Read the model definition and answer for the solid it produces. Units are mm, in the model's axes. Face numbers are marked on the shaded views. A direction names the side the tool comes from. Give positions to 0.01 mm unless a question says otherwise; leave off trailing zeros. Write each loop counter-clockwise with the first axis right and the second up, starting at its lowest first coordinate (ties: lowest second). Pieces come first, ordered by that corner, then holes. Notation, with made-up numbers: M -32.5,5 L -18.5,5 A23 ccw -18.5,18 Z; hole C 37.25,25.25 d11. An arc over 180 degrees is marked long. Put each result on its own line as item: value.
from build123d import *

# Parameters (mm, degrees)
ENL_V_START             = -10
ENL_V_MAT_EXTRU_1_DEPTH = 10


with BuildPart() as part:
    # Esquisse1 → R_volution1 (revolve)
    with BuildSketch(Plane.XY, mode=Mode.PRIVATE) as r_volution1_sk:
        with BuildLine():
            Line((38.667823993, 0), (38.667823993, 1.585))
            Line((38.667823993, 1.585), (36.667823993, 1.585))
            Line((36.667823993, 1.585), (33.667823993, 4.585))
            Line((33.667823993, 4.585), (33.667823993, 7.5))
            Line((33.667823993, 7.5), (40.667823993, 7.5))
            Line((40.667823993, 7.5), (40.667823993, 1.5))
            Line((40.667823993, 1.5), (47.667823993, 1.5))
            Line((47.667823993, 1.5), (47.667823993, 7))
            Line((47.667823993, 7), (49.167823993, 7))
            Line((49.167823993, 7), (49.167823993, 1.5))
            Line((49.167823993, 1.5), (49.667823993, 1.5))
            Line((49.667823993, 1.5), (49.667823993, 7))
            Line((49.667823993, 7), (50.667823993, 7))
            Line((50.667823993, 7), (50.667823993, 6))
            add(Edge.make_bspline(
                [(50.667823993, 6), (54.792010738, 6.082824703), (58.901540934, 4.911130099), (62.781307834, 2.984328023)],
                knots=[0, 0, 0, 0, 1, 1, 1, 1], degree=3))
            add(Edge.make_bspline(
                [(62.781307834, 2.984328023), (64.265948318, 2.24701353), (65.473917032, 1.727596368), (65.667823993, 0)],
                knots=[0, 0, 0, 0, 1, 1, 1, 1], degree=3))
            Line((65.667823993, 0), (38.667823993, 0))
        make_face()
    revolve(r_volution1_sk.sketch.rotate(Axis((0, 0, 0), (1, 0, 0)), 90), axis=Axis((0, 0, 0), (1, 0, 0)))

    # Esquisse2 → Enl_v. mat.-Extru.1 (cut)
    with BuildSketch(Plane.ZY.offset(-33.667823993).offset(ENL_V_START)):
        with BuildLine():
            Line((-3, 5), (-3, 6.873863542))
            ThreePointArc((-3, 6.873863542), (-5.303300859, 5.303300859), (-6.873863542, 3))
            Line((-6.873863542, 3), (-5, 3))
            ThreePointArc((-5, 3), (-3.585786438, 3.585786438), (-3, 5))
        make_face()
        with BuildLine():
            ThreePointArc((6.873863542, 3), (5.303300859, 5.303300859), (3, 6.873863542))
            Line((3, 6.873863542), (3, 5))
            ThreePointArc((3, 5), (3.585786438, 3.585786438), (5, 3))
            Line((5, 3), (6.873863542, 3))
        make_face()
        with BuildLine():
            ThreePointArc((3, -6.873863542), (5.303300859, -5.303300859), (6.873863542, -3))
            Line((6.873863542, -3), (5, -3))
            ThreePointArc((5, -3), (3.585786438, -3.585786438), (3, -5))
            Line((3, -5), (3, -6.873863542))
        make_face()
        with BuildLine():
            Line((-5, -3), (-6.873863542, -3))
            ThreePointArc((-6.873863542, -3), (-5.303300859, -5.303300859), (-3, -6.873863542))
            Line((-3, -6.873863542), (-3, -5))
            ThreePointArc((-3, -5), (-3.585786438, -3.585786438), (-5, -3))
        make_face()
    extrude(amount=ENL_V_MAT_EXTRU_1_DEPTH, mode=Mode.SUBTRACT)


solid = part.part
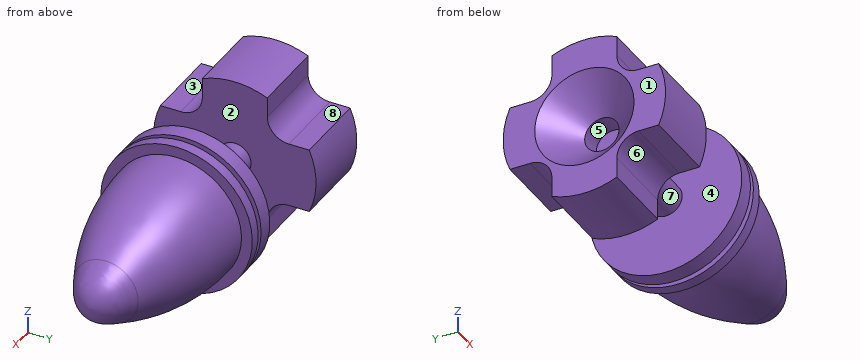
(1) Which of the six approach directions +Z, -Z, +X, -X, +Y, -Y give full straight-line access (tool end or side, diameter ignored) to the marked faces 5, 6, 7 and 8?
Result:
face 5: -X
face 6: -Z, -X, -Y
face 7: none
face 8: +Z, -X, +Y
(2) Section B-B on z = 3.5 is taken. Give the number of separate pieces and of enclosed holes in the cut face, and give its area (3 significant figures).
Result:
separate pieces: 3
enclosed holes: 0
area: 160 mm²
(3) Given pin 1 Ø6 at (x, y) = (38, -3) entering from +Z; pin 2 Ø0.6 at (x, z) = (36, 6.5) entering from -Y; pin 3 Ø8 at (x, z) = (56, 1.5) entering from -Y; pin 4 Ø4 at (y, z) = (-1, 1) entering from -X, each flat-ended and moving along its own axis, determine where each tip first touches the part or whether it passes through.
Result:
pin 1: stops at z = 7.5
pin 2: stops at y = -3
pin 3: stops at y = -5.97
pin 4: stops at x = 34.84
(4) Straight lines are drawn through the part: line 1 along X through (y, z) = (3, 2.75); line 2 along Y through (x, z) = (37.8, 0) (3 decimals); line 3 along X through (y, z) = (2, -1.75). For each, find the intervals that lie inside material, in ascending order. Write a range as from..to.
Result:
line 1: x = 34.18..40.67, 47.67..49.17, 49.67..60.37
line 2: y = -7.5..-1.585, 1.585..7.5
line 3: x = 35.6..40.67, 47.67..49.17, 49.67..63.44
(5) Section C-C on x = 50 is taken. Determine the outline of the cut face in (y, z), and give its area (3 significant figures).
Result:
outline: C 0,0 d14
area: 154 mm²
(6) For a pull along X with two mould halves and no side action, classify the marked faces 1, 2, 3 and 4 as +X half, -X half, draft (parallel to the pull), parting line (faces both ways), or undercut.
Result:
face 1: -X half
face 2: undercut
face 3: draft
face 4: undercut
(7) Section A-A on x = 46 is taken. Determine the outline of the cut face in (y, z), and give its area (3 significant figures).
Result:
outline: C 0,0 d3
area: 7.07 mm²
